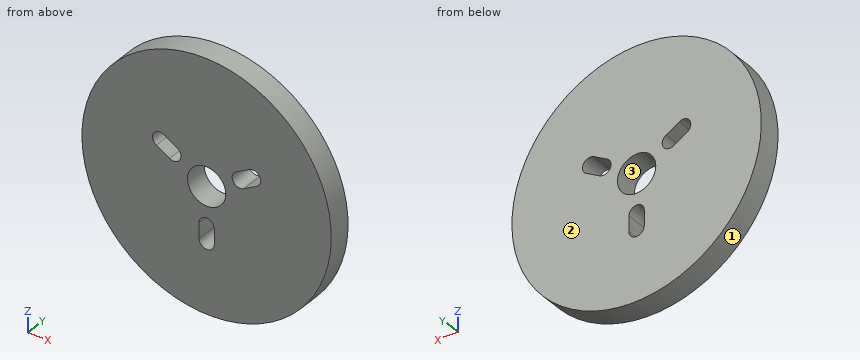
from build123d import *

# Parameters (mm, degrees)
SKETCH1_R           = 32.5
SKETCH1_R_2         = 5
BOSS_EXTRUDE1_DEPTH = 6


with BuildPart() as part:
    # Sketch1 → Boss-Extrude1 (new body)
    with BuildSketch(Plane(origin=(0, 0, 0), x_dir=(1, 0, 0), z_dir=(0, 1, 0))):
        with Locations(Location((0, 0, 0), (0, 0, 270))):
            Circle(SKETCH1_R)
        with Locations(Location((0, 0, 0), (0, 0, 270))):
            Circle(SKETCH1_R_2, mode=Mode.SUBTRACT)
        with BuildLine():
            Line((-2, 10), (-2, 14))
            ThreePointArc((-2, 14), (0, 16), (2, 14))
            Line((2, 14), (2, 10))
            ThreePointArc((2, 10), (0, 8), (-2, 10))
        make_face(mode=Mode.SUBTRACT)
        with BuildLine():
            Line((9.660254038, -3.267949192), (13.124355653, -5.267949192))
            ThreePointArc((13.124355653, -5.267949192), (13.856406461, -8), (11.124355653, -8.732050808))
            Line((11.124355653, -8.732050808), (7.660254038, -6.732050808))
            ThreePointArc((7.660254038, -6.732050808), (6.92820323, -4), (9.660254038, -3.267949192))
        make_face(mode=Mode.SUBTRACT)
        with BuildLine():
            Line((-7.660254038, -6.732050808), (-11.124355653, -8.732050808))
            ThreePointArc((-11.124355653, -8.732050808), (-13.856406461, -8), (-13.124355653, -5.267949192))
            Line((-13.124355653, -5.267949192), (-9.660254038, -3.267949192))
            ThreePointArc((-9.660254038, -3.267949192), (-6.92820323, -4), (-7.660254038, -6.732050808))
        make_face(mode=Mode.SUBTRACT)
    extrude(amount=BOSS_EXTRUDE1_DEPTH)


solid = part.part
The model under review builds one solid part; all positions refer to its coordinate system, in mm. Face numbers are marked on the shaded views. Give positions to 0.01 mm unless a question says otherwise; leave off trailing zeros. Loops run counter-clockwise (first coordinate to the right, second up) from the corner with the lowest first, then second, coordinate; pieces in that order, holes last. Notation, with made-up numbers: (-35, -33) -> (-7, -33) arc R22 ccw to (-7, -7) -> close; hole circle Ø7 at (-14, 78.25). An arc over 180 degrees is marked (long way). Put each result on its own line as item: value. Start each with the question number.
1. Wall thickness on probe 1 along X at (y, z) = (1, 0); probe 2 along Z at (x, y) = (10.5, 1.25); probe 3 along Z at (x, y) = (-7, 3.95): over which ranges is each line inside the solid? List them lowest first.
2. Clearance check with flat-ended pins moving along their axes: P1, Ø1, axis at x = -20.5, y = 2, coming from the -Z side; P2, Ø3, axis at y = 0.5, z = -5.5, coming from the +X side; P3, Ø2, axis at y = 3.5, z = -12, coming from the -X side. State where each tip first meets the part, or that it passes through.
3. We need section C-C on x = 0. State the section outline as (y, z) points, then the cut area to 3 significant figures.
4. We need section A-A on y = 4.2. State the section outline as (x, z) points.
5. Mouldability with a two-part tool opening along X and no side actions: class the marked faces 1, 2 and 3 as released by +X, released by -X, zero draft, split by the parting line, or undercut.
6. We need section B-B on z = 0. State the section outline as (x, y) points, then the cut area to 3 significant figures.
7. We need section D-D on x = -21.5. State the section outline as (y, z) points, then the cut area to 3 significant figures.
Determined:
1. probe 1: -32.5 to -5, 5 to 32.5
1. probe 2: -30.76 to 3.75, 8.37 to 30.76
1. probe 3: -31.74 to 3.88, 6.12 to 31.74
2. P1: z = -25.62
2. P2: x = 32.25
2. P3: x = -30.58
3. outline: (0, -32.5) -> (6, -32.5) -> (6, -16) -> (0, -16) -> close; (0, -8) -> (6, -8) -> (6, -5) -> (0, -5) -> close; (0, 5) -> (6, 5) -> (6, 32.5) -> (0, 32.5) -> close
3. area: 282 mm^2
4. outline: circle Ø65 at (0, 0); hole (-13.12, 5.27) -> (-9.66, 3.27) arc R2 ccw to (-7.66, 6.73) -> (-11.12, 8.73) arc R2 ccw to start; hole circle Ø10 at (0, 0); hole (-2, -14) arc R2 ccw to (2, -14) -> (2, -10) arc R2 ccw to (-2, -10) -> close; hole (7.66, 6.73) arc R2 ccw to (9.66, 3.27) -> (13.12, 5.27) arc R2 ccw to (11.12, 8.73) -> close
5. face 1: split by the parting line
5. face 2: zero draft
5. face 3: undercut
6. outline: (-32.5, 0) -> (-5, 0) -> (-5, 6) -> (-32.5, 6) -> close; (5, 0) -> (32.5, 0) -> (32.5, 6) -> (5, 6) -> close
6. area: 330 mm^2
7. outline: (0, -24.37) -> (6, -24.37) -> (6, 24.37) -> (0, 24.37) -> close
7. area: 292 mm^2
